Design review of the part shown in the three views and the two pictorial views. Dimensions are in mm from the part's minimum x, y and z. A direction names the side the tool comes from. Coordinates: 2 decimals unless noted, no trailing zeros. Write each loop counter-clockwise with the first axis right and the second up, starting at its lowest first coordinate (ties: lowest second). Pieces come first, ordered by that corner, then holes. Notation, with made-up numbers: (13, 51.25) -> (53, 51.25) arc R15 cw to (53, 64.25) -> close; hole circle Ø1 at (14, -16). An arc over 180 degrees is marked (long way). Write item = value, one per line. Start each with the question number.
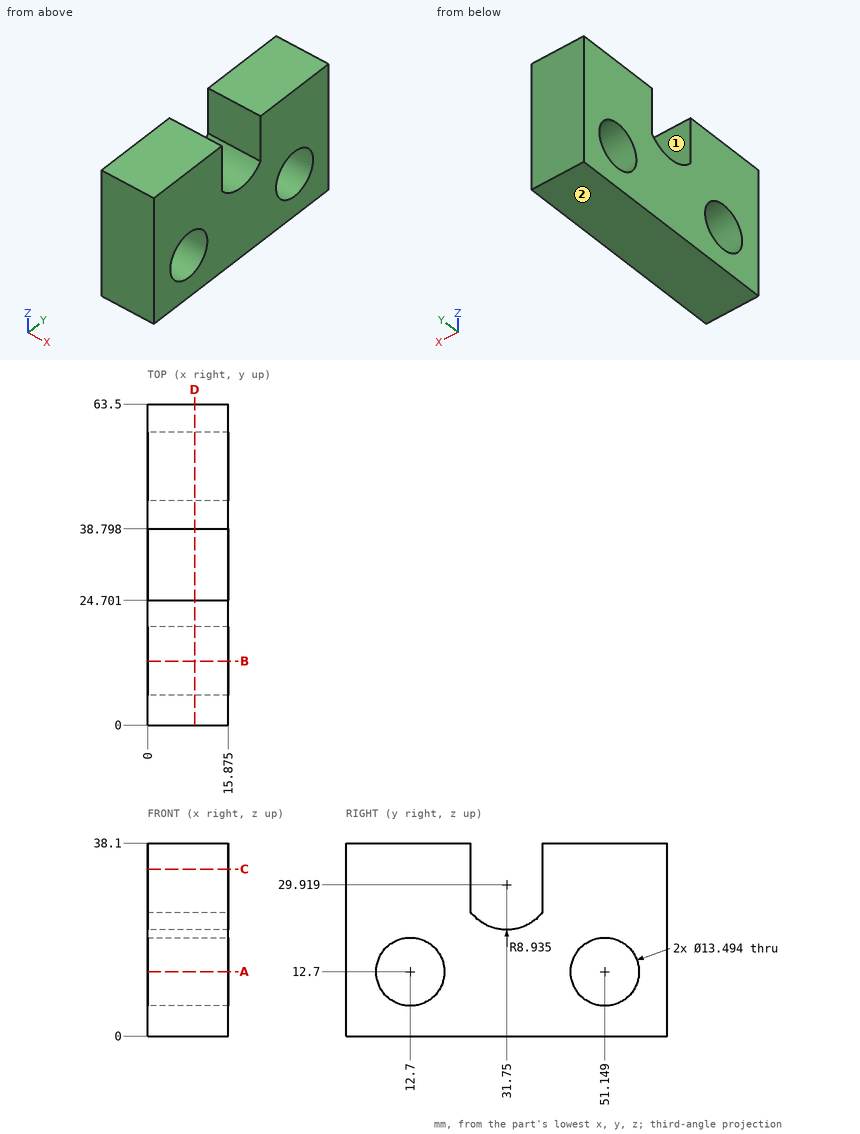
(1) For line 1 (Y direction, x = 9.5, z = 12.7); line 2 (Y direction, x = 1.75, z = 30); line 3 (Y direction, x = 5.75, z = 8.5), list the stretches that pass through material, from the lowest coordinate up.
(2) Take a section at D-D, the plane x = 9.25. Count the separate pieces of the cut face and the enclosed holes in it, then the cut area to 3 significant figures.
(3) For the marked faces 1 and 2, list the 3-axis set-ups (+Z, -Z, +X, -X, +Y, -Y) from which the entire face can be reached by the end or side of a thin tool; tool diameter is ignored.
(4) Take a section at B-B, the plane y = 12.7. State the section outline as (x, z) points (1 decimal).
(5) Take a section at A-A, the plane z = 12.7. State the section outline as (x, y) points (1 decimal).
(6) Take a section at C-C, the plane z = 33. State the section outline as (x, y) points (1 decimal), then the cut area to 3 significant figures.
Report:
q1.line_1 = 0 to 5.95, 19.45 to 44.4, 57.9 to 63.5
q1.line_2 = 0 to 24.7, 38.8 to 63.5
q1.line_3 = 0 to 7.42, 17.98 to 45.87, 56.43 to 63.5
q2.separate_pieces = 1
q2.enclosed_holes = 2
q2.area = 1,910 mm2
q3.face_1 = +Z, +X, -X
q3.face_2 = -Z, +X, -X, +Y, -Y
q4.outline = (0, 0) -> (15.9, 0) -> (15.9, 6) -> (0, 6) -> close; (0, 19.4) -> (15.9, 19.4) -> (15.9, 38.1) -> (0, 38.1) -> close
q5.outline = (0, 0) -> (15.9, 0) -> (15.9, 6) -> (0, 6) -> close; (0, 19.4) -> (15.9, 19.4) -> (15.9, 44.4) -> (0, 44.4) -> close; (0, 57.9) -> (15.9, 57.9) -> (15.9, 63.5) -> (0, 63.5) -> close
q6.outline = (0, 0) -> (15.9, 0) -> (15.9, 24.7) -> (0, 24.7) -> close; (0, 38.8) -> (15.9, 38.8) -> (15.9, 63.5) -> (0, 63.5) -> close
q6.area = 784 mm2
